Design review of the part shown in the three views and the two pictorial views. Dimensions are in mm from the part's minimum x, y and z. A direction names the side the tool comes from. Give positions to 0.01 mm unless a question says otherwise; leave off trailing zeros. Loops run counter-clockwise (first coordinate to the right, second up) from the corner with the lowest first, then second, coordinate; pieces in that order, holes last. Notation, with made-up numbers: (6.25, 59.25) -> (48.25, 59.25) arc R20 ccw to (48.25, 87.25) -> close; hole circle Ø11 at (-23.75, -17.75). An arc over 180 degrees is marked (long way). One line per question, with ' | ' between items. Start each with the question number.
(1) Consider section B-B (x = 29.75). Write out the cut boundary in (y, z), and give its area (3 significant figures).
(2) Wall thickness on probe 1 along Y at (x, z) = (2.25, 18.9); probe 2 along Z at (x, y) = (28, 5); probe 3 along X at (y, z) = (6.15, 18.8): over which ranges is each line inside the solid? List them lowest first.
(3) Consider section C-C (z = 19). Write out the cut boundary in (x, y).
(4) Insertion check: P1, Ø4, axis at y = 6.5, z = 9, coming from the +X side; P2, Ø2, axis at y = 10, z = 8.5, coming from the -X side; P3, Ø5, axis at x = 3.5, y = 8.5, coming from the +Z side. Each pin has a flat end and moves straight along its axis. Give the tip position at first contact, or say it passes through.
(5) Consider section D-D (y = 3.25). Write out the cut boundary in (x, z).
(6) Tool access review of the marked faces 1, 2, 3 and 4: name each direction out of +Z, -Z, +X, -X, +Y, -Y from which nothing blocks a thin tool from reaching the whole face with its end or side.
(7) Consider section A-A (x = 21). Write out the cut boundary in (y, z).
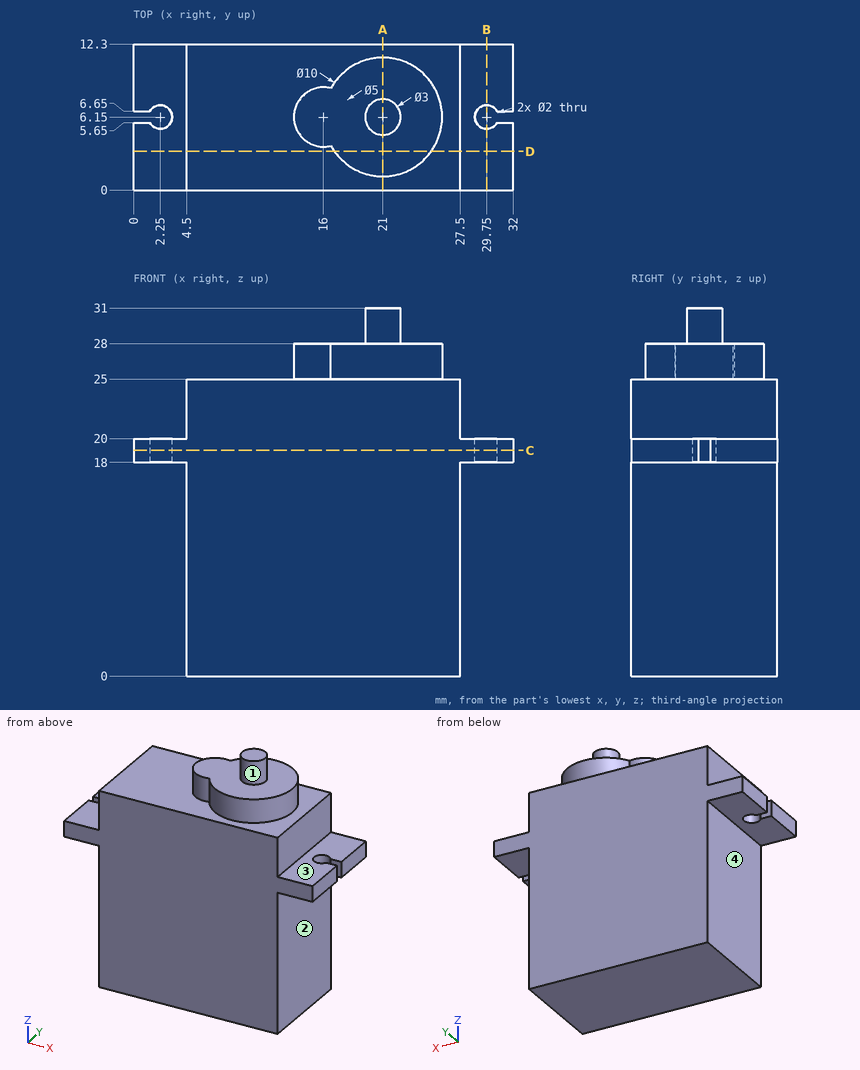
A:
1) outline: (0, 18) -> (5.15, 18) -> (5.15, 20) -> (0, 20) -> close; (7.15, 18) -> (12.3, 18) -> (12.3, 20) -> (7.15, 20) -> close | area: 20.6 mm^2
2) probe 1: y = 0 to 5.15, 7.15 to 12.3 | probe 2: z = 18 to 20 | probe 3: x = 3.25 to 28.75
3) outline: (0, 0) -> (32, 0) -> (32, 5.65) -> (30.62, 5.65) arc R1 cw (long way) to (30.62, 6.65) -> (32, 6.65) -> (32, 12.3) -> (0, 12.3) -> (0, 6.65) -> (1.38, 6.65) arc R1 cw (long way) to (1.38, 5.65) -> (0, 5.65) -> close
4) P1: stops at x = 27.5 | P2: stops at x = 4.5 | P3: stops at z = 25
5) outline: (0, 18) -> (4.5, 18) -> (4.5, 0) -> (27.5, 0) -> (27.5, 18) -> (32, 18) -> (32, 20) -> (27.5, 20) -> (27.5, 25) -> (25.07, 25) -> (25.07, 28) -> (16.93, 28) -> (16.93, 25) -> (4.5, 25) -> (4.5, 20) -> (0, 20) -> close
6) face 1: +Z | face 2: -Z, +X, +Y, -Y | face 3: +Z, +X, +Y, -Y | face 4: -Z, -X, +Y, -Y
7) outline: (0, 0) -> (12.3, 0) -> (12.3, 25) -> (11.15, 25) -> (11.15, 28) -> (7.65, 28) -> (7.65, 31) -> (4.65, 31) -> (4.65, 28) -> (1.15, 28) -> (1.15, 25) -> (0, 25) -> close
